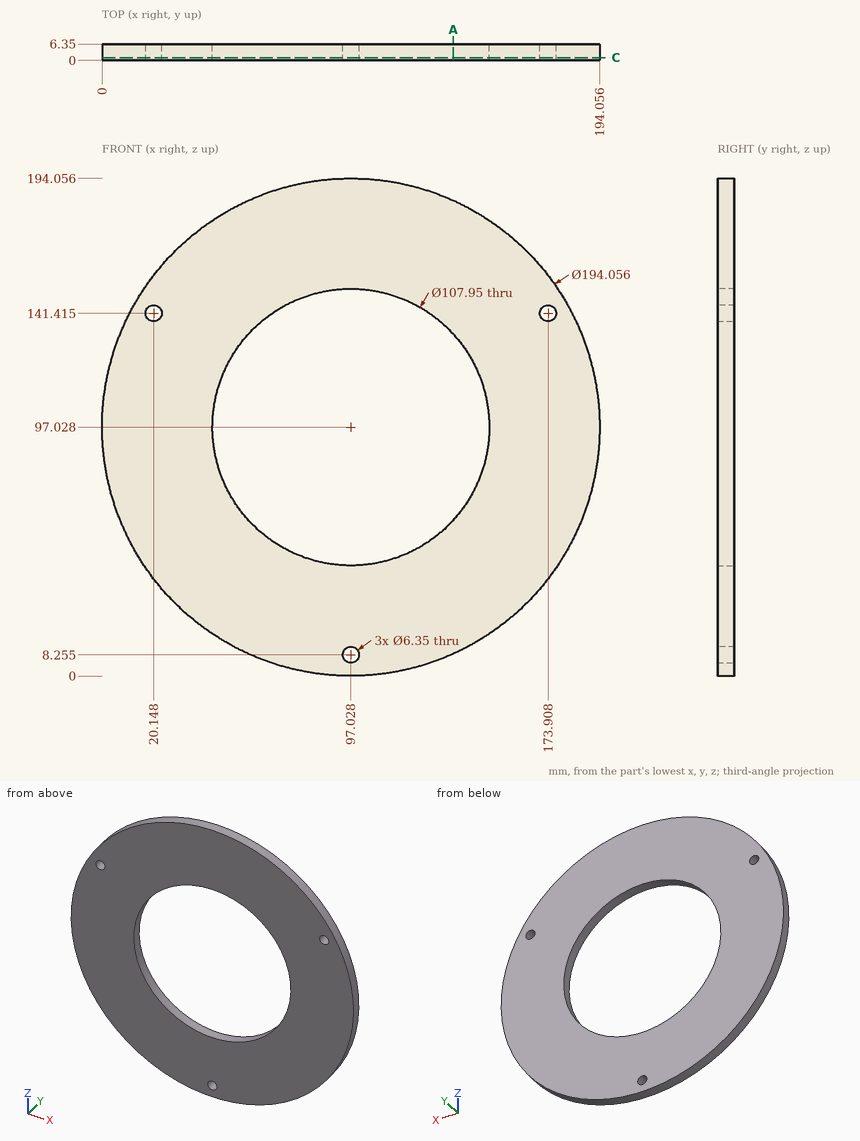
The figure shows three views and two pictorial views of one solid part (mm, origin at its lowest corner). Answer the questions. Give positions to 0.01 mm unless a question says otherwise; leave off trailing zeros. Loops run counter-clockwise (first coordinate to the right, second up) from the corner with the lowest first, then second, coordinate; pieces in that order, holes last. Notation, with made-up numbers: (-35.5, -33) -> (20.5, -33) arc R19 cw to (20.5, -17) -> close; hole circle Ø1 at (11.5, 0.25). An arc over 180 degrees is marked (long way). Use a Markdown table: item, result. Add a question column.
1. Section A-A on x = 137 is taken. Determine the outline of the cut face in (y, z).
2. Find the intervals of material crossed by probe 1 along Z at (x, y) = (128, 5) (1 decimal); probe 2 along Z at (x, y) = (121.5, 4) (1 decimal); probe 3 along X at (y, z) = (0.5, 132) (1 decimal), in increasing order.
3. Flat-ended cylindrical pins translate along their axes: pin 1 Ø3 at (x, y) = (100.5, 1) entering from -Z; pin 2 Ø10 at (x, z) = (97.028, 8.255) entering from +Y; pin 3 Ø2 at (x, y) = (40, 1) entering from -Z; pin 4 Ø1 at (y, z) = (4.5, 70) entering from +X. Find the tip coordinate at first contact, or state that the pin passes through.
4. Section C-C on y = 1 is taken. State how many separate pieces and enclosed holes the cut face has, and give its area (3 significant figures).
Results below:
| question | item | result |
|---|---|---|
| 1 | outline | (0, 8.62) -> (6.35, 8.62) -> (6.35, 60.76) -> (0, 60.76) -> close; (0, 133.3) -> (6.35, 133.3) -> (6.35, 185.44) -> (0, 185.44) -> close |
| 2 | probe 1 | z = 5.1 to 52.8, 141.2 to 189 |
| 2 | probe 2 | z = 3.1 to 48.9, 145.1 to 190.9 |
| 2 | probe 3 | x = 6.5 to 55.9, 138.1 to 187.5 |
| 3 | pin 1 | stops at z = 0.02 |
| 3 | pin 2 | stops at y = 6.35 |
| 3 | pin 3 | stops at z = 17.81 |
| 3 | pin 4 | stops at x = 190.36 |
| 4 | separate pieces | 1 |
| 4 | enclosed holes | 4 |
| 4 | area | 20,300 mm^2 |
